from build123d import *

# Parameters (mm, degrees)
BOSS_EXTRUDE1_DEPTH = 3


with BuildPart() as part:
    # Sketch1 → Boss-Extrude1 (new body)
    with BuildSketch(Plane.XY):
        with BuildLine():
            Line((-176.261287631, -146.790125913), (-174.178854352, -176.465678255))
            ThreePointArc((-174.178854352, -176.465678255), (-174.10743246, -176.805459554), (-173.946658522, -177.113199961))
            ThreePointArc((-173.946658522, -177.113199961), (-165.987154225, -184.643491087), (-155.766014333, -188.591565607))
            ThreePointArc((-155.766014333, -188.591565607), (-155.419681283, -188.604453413), (-155.08275986, -188.523233763))
            Line((-155.08275986, -188.523233763), (-127.359223318, -177.660950501))
            ThreePointArc((-127.359223318, -177.660950501), (-125.666782112, -177.423691901), (-124.049456606, -177.975875826))
            Line((-124.049456606, -177.975875826), (-122.862735706, -178.725113106))
            ThreePointArc((-122.862735706, -178.725113106), (-121.236507239, -181.027562815), (-121.714667864, -183.805557795))
            Line((-121.714667864, -183.805557795), (-125.240247105, -189.389741443))
            ThreePointArc((-125.240247105, -189.389741443), (-127.862246775, -192.636349191), (-131.161557479, -195.191714728))
            ThreePointArc((-131.161557479, -195.191714728), (-140.433747596, -199.259536064), (-150.43809188, -200.819592292))
            Line((-150.43809188, -200.819592292), (-177.583691953, -201.507185822))
            ThreePointArc((-177.583691953, -201.507185822), (-179.816644976, -200.815129336), (-181.172145987, -198.910493309))
            Line((-181.172145987, -198.910493309), (-189.006171765, -172.910792767))
            ThreePointArc((-189.006171765, -172.910792767), (-190.489642304, -165.396715762), (-190.485324726, -157.737602274))
            ThreePointArc((-190.485324726, -157.737602274), (-189.596958817, -153.660084628), (-187.793276628, -149.89683142))
            Line((-187.793276628, -149.89683142), (-184.267697387, -144.312647772))
            ThreePointArc((-184.267697387, -144.312647772), (-181.965247678, -142.686419305), (-179.187252699, -143.16457993))
            Line((-179.187252699, -143.16457993), (-177.969064462, -143.933684141))
            ThreePointArc((-177.969064462, -143.933684141), (-176.774137848, -145.158008999), (-176.261287631, -146.790125913))
        make_face()
        with BuildLine():
            Line((-177.401483744, -146.870137307), (-175.319050465, -176.54568965))
            ThreePointArc((-175.319050465, -176.54568965), (-175.183348871, -177.191274117), (-174.877878388, -177.775980891))
            ThreePointArc((-174.877878388, -177.775980891), (-166.597350632, -185.60998441), (-155.963970787, -189.717293035))
            ThreePointArc((-155.963970787, -189.717293035), (-155.305937992, -189.741779868), (-154.665787288, -189.587462533))
            Line((-154.665787288, -189.587462533), (-126.942250746, -178.72517927))
            ThreePointArc((-126.942250746, -178.72517927), (-125.775049914, -178.56155265), (-124.659653013, -178.94236915))
            Line((-124.659653013, -178.94236915), (-123.472932113, -179.69160643))
            ThreePointArc((-123.472932113, -179.69160643), (-122.351395239, -181.279502781), (-122.681161188, -183.195361388))
            Line((-122.681161188, -183.195361388), (-126.206740429, -188.779545035))
            ThreePointArc((-126.206740429, -188.779545035), (-128.66220108, -191.819941137), (-131.751952653, -194.21299999))
            ThreePointArc((-131.751952653, -194.21299999), (-140.75407898, -198.162341093), (-150.467034596, -199.67695879))
            Line((-150.467034596, -199.67695879), (-177.612634669, -200.36455232))
            ThreePointArc((-177.612634669, -200.36455232), (-179.146576312, -199.889139604), (-180.077746571, -198.580737463))
            Line((-180.077746571, -198.580737463), (-187.911772349, -172.581036921))
            ThreePointArc((-187.911772349, -172.581036921), (-189.352035008, -165.285816528), (-189.347843185, -157.849784016))
            ThreePointArc((-189.347843185, -157.849784016), (-188.515902755, -154.031254117), (-186.826783305, -150.507027827))
            Line((-186.826783305, -150.507027827), (-183.301204063, -144.922844179))
            ThreePointArc((-183.301204063, -144.922844179), (-181.713307713, -143.801307305), (-179.797449106, -144.131073254))
            Line((-179.797449106, -144.131073254), (-178.579260869, -144.900177465))
            ThreePointArc((-178.579260869, -144.900177465), (-177.755173549, -145.744539435), (-177.401483744, -146.870137307))
        make_face(mode=Mode.SUBTRACT)
    extrude(amount=BOSS_EXTRUDE1_DEPTH)


solid = part.part
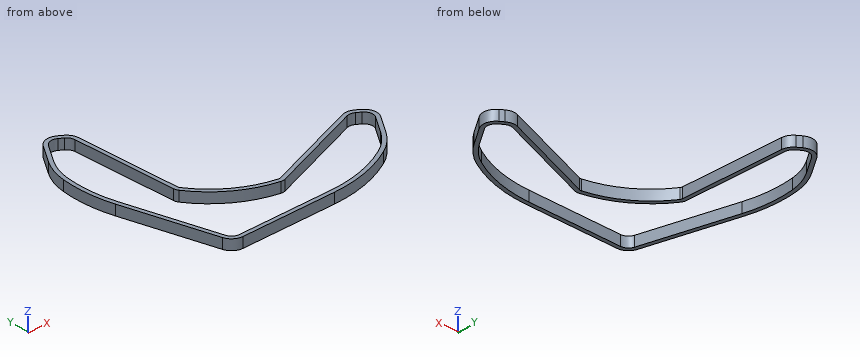
Build history of the part. All positions in model axes, mm. Round coordinates to 2 decimals unless told otherwise and drop trailing zeros. Loops run counter-clockwise (first coordinate to the right, second up) from the corner with the lowest first, then second, coordinate; pieces in that order, holes last. Notation, with made-up numbers: (9.5, -18.5) -> (41.5, -18.5) arc R15 ccw to (41.5, 2.5) -> close; hole circle Ø11 at (26.5, 57.25). An arc over 180 degrees is marked (long way). Answer in a Markdown table with one row per item.
Item 1: Saw through at B-B (y = -182). Write the cut outline in (x, z), and give its area (3 significant figures).
Answers below:
| item | result |
|---|---|
| outline | (-186.27, 0) -> (-185.07, 0) -> (-185.07, 3) -> (-186.27, 3) -> close; (-171.22, 0) -> (-169.53, 0) -> (-169.53, 3) -> (-171.22, 3) -> close; (-138.43, 0) -> (-135.3, 0) -> (-135.3, 3) -> (-138.43, 3) -> close; (-122.29, 0) -> (-121.15, 0) -> (-121.15, 3) -> (-122.29, 3) -> close |
| area | 21.5 mm² |
Item 2: Saw through at C-C (x = -143). Write the cut outline in (y, z), and give its area (3 significant figures).
Answers below:
| item | result |
|---|---|
| outline | (-199.92, 0) -> (-198.74, 0) -> (-198.74, 3) -> (-199.92, 3) -> close; (-185.02, 0) -> (-183.79, 0) -> (-183.79, 3) -> (-185.02, 3) -> close |
| area | 7.20 mm² |
Item 3: Drill centre lines: L1, parallel to X at y = -163.5, z = 1.15; L2, parallel to X at y = -158.5, z = 1.5; L3, parallel to Y at x = -172, z = 2.1. Where is each one in solid material? Low to high. Write a range as [from, to].
Answers below:
| item | result |
|---|---|
| L1 | x = [-190.63, -189.48], [-176.23, -175.09] |
| L2 | x = [-190.55, -189.41], [-176.59, -175.44] |
| L3 | y = [-201.37, -200.22], [-181.23, -179.55] |
Item 4: Saw through at A-A (y = -161). Write the cut outline in (x, z).
Answers below:
| item | result |
|---|---|
| outline | (-190.67, 0) -> (-189.53, 0) -> (-189.53, 3) -> (-190.67, 3) -> close; (-176.41, 0) -> (-175.26, 0) -> (-175.26, 3) -> (-176.41, 3) -> close |
